from build123d import *
from OCP.BRepFilletAPI import BRepFilletAPI_MakeChamfer

# Parameters (mm, degrees)
EXTRUDE_1_DEPTH     = 60
FILLET_1_R          = 5
CUT_EXTRUDE_1_DEPTH = 5.9
CHAMFER_1_SIZE      = 0.5
CHAMFER_1_SIZE2     = 0.355637567
CHAMFER_1_SIZE2_2   = 0.356604189
SKETCH_6_R          = 2.85
CUT_EXTRUDE_2_DEPTH = 0.1
SKETCH_7_R          = 2.5
CUT_EXTRUDE_3_DEPTH = 75.215901261


with BuildPart() as part:
    # 草图1 → 凸台-拉伸1 (new body)
    with BuildSketch(Plane.XY):
        Polygon((0, 0), (42, 0), (42, 10), (40.535898385, 12), (40, 10), (38.535898385, 12), (38, 10), (36.535898385, 12), (36, 10), (34.535898385, 12), (34, 10), (32.535898385, 12), (32, 10), (30.535898385, 12), (30, 10), (28.535898385, 12), (28, 10), (26.535898385, 12), (26, 10), (24.535898385, 12), (24, 10), (22.535898385, 12), (22, 10), (20.535898385, 12), (20, 10), (18.535898385, 12), (18, 10), (16.535898385, 12), (16, 10), (14.535898385, 12), (14, 10), (12.535898385, 12), (12, 10), (10.535898385, 12), (10, 10), (8.51763809, 11.931851653), (8, 10), (6, 12), (0, 12), align=None)
    extrude(amount=EXTRUDE_1_DEPTH)

    # 圆角1
    fillet_1_edges = [part.edges().sort_by_distance(p)[0] for p in [
        (42, 5, 0),
        (42, 5, 60),
    ]]
    fillet(fillet_1_edges, radius=FILLET_1_R)

    # 草图2 → 切除-拉伸1 (cut)
    with BuildSketch(Plane.ZY):
        with BuildLine():
            ThreePointArc((32.9, 12), (32.050609665, 9.949390335), (30, 9.1))
            Line((30, 9.1), (30, 0))
            Line((30, 0), (39, 0))
            Line((39, 0), (39, 12))
            Line((39, 12), (32.9, 12))
        make_face()
        with BuildLine():
            Line((30, 0), (30, 9.1))
            ThreePointArc((30, 9.1), (27.949390335, 9.949390335), (27.1, 12))
            Line((27.1, 12), (21, 12))
            Line((21, 12), (21, 0))
            Line((21, 0), (30, 0))
        make_face()
        with BuildLine():
            Line((32.9, 12), (30, 12))
            Line((30, 12), (30, 9.1))
            ThreePointArc((30, 9.1), (32.050609665, 9.949390335), (32.9, 12))
        make_face()
        with BuildLine():
            Line((30, 9.1), (30, 12))
            Line((30, 12), (27.1, 12))
            ThreePointArc((27.1, 12), (27.949390335, 9.949390335), (30, 9.1))
        make_face()
    extrude(amount=-CUT_EXTRUDE_1_DEPTH, mode=Mode.SUBTRACT)

    # 倒角1: one chamfer whose edges measure the first distance from different faces: ONE call of the kernel's chamfer builder (chamfer() names one face for all edges)
    chamfer_1_edges_1 = [part.edges().sort_by_distance(p)[0] for p in [
        (40.535898385, 12, 30),
    ]]
    chamfer_1_side_1 = [part.faces().sort_by_distance(p)[0] for p in [
        (40.267229154, 10.997312779, 30),
    ]]
    chamfer_1_edges_2 = [part.edges().sort_by_distance(p)[0] for p in [
        (38.535898385, 12, 30),
    ]]
    chamfer_1_side_2 = [part.faces().sort_by_distance(p)[0] for p in [
        (38.267738685, 10.999214377, 30),
    ]]
    chamfer_1_edges_3 = [part.edges().sort_by_distance(p)[0] for p in [
        (36.535898385, 12, 30),
    ]]
    chamfer_1_side_3 = [part.faces().sort_by_distance(p)[0] for p in [
        (36.267949192, 11, 30),
    ]]
    chamfer_1_edges_4 = [part.edges().sort_by_distance(p)[0] for p in [
        (34.535898385, 12, 30),
    ]]
    chamfer_1_side_4 = [part.faces().sort_by_distance(p)[0] for p in [
        (34.267949192, 11, 30),
    ]]
    chamfer_1_edges_5 = [part.edges().sort_by_distance(p)[0] for p in [
        (32.535898385, 12, 30),
    ]]
    chamfer_1_side_5 = [part.faces().sort_by_distance(p)[0] for p in [
        (32.267949192, 11, 30),
    ]]
    chamfer_1_edges_6 = [part.edges().sort_by_distance(p)[0] for p in [
        (30.535898385, 12, 30),
    ]]
    chamfer_1_side_6 = [part.faces().sort_by_distance(p)[0] for p in [
        (31.267949192, 11, 30),
    ]]
    chamfer_1_edges_7 = [part.edges().sort_by_distance(p)[0] for p in [
        (28.535898385, 12, 30),
    ]]
    chamfer_1_side_7 = [part.faces().sort_by_distance(p)[0] for p in [
        (29.267949192, 11, 30),
    ]]
    chamfer_1_edges_8 = [part.edges().sort_by_distance(p)[0] for p in [
        (26.535898385, 12, 30),
    ]]
    chamfer_1_side_8 = [part.faces().sort_by_distance(p)[0] for p in [
        (27.267949192, 11, 30),
    ]]
    chamfer_1_edges_9 = [part.edges().sort_by_distance(p)[0] for p in [
        (24.535898385, 12, 30),
    ]]
    chamfer_1_side_9 = [part.faces().sort_by_distance(p)[0] for p in [
        (25.267949192, 11, 30),
    ]]
    chamfer_1_edges_10 = [part.edges().sort_by_distance(p)[0] for p in [
        (22.535898385, 12, 30),
    ]]
    chamfer_1_side_10 = [part.faces().sort_by_distance(p)[0] for p in [
        (23.267949192, 11, 30),
    ]]
    chamfer_1_edges_11 = [part.edges().sort_by_distance(p)[0] for p in [
        (20.535898385, 12, 30),
    ]]
    chamfer_1_side_11 = [part.faces().sort_by_distance(p)[0] for p in [
        (21.267949192, 11, 30),
    ]]
    chamfer_1_edges_12 = [part.edges().sort_by_distance(p)[0] for p in [
        (18.535898385, 12, 30),
    ]]
    chamfer_1_side_12 = [part.faces().sort_by_distance(p)[0] for p in [
        (19.267949192, 11, 30),
    ]]
    chamfer_1_edges_13 = [part.edges().sort_by_distance(p)[0] for p in [
        (16.535898385, 12, 30),
    ]]
    chamfer_1_side_13 = [part.faces().sort_by_distance(p)[0] for p in [
        (17.267949192, 11, 30),
    ]]
    chamfer_1_edges_14 = [part.edges().sort_by_distance(p)[0] for p in [
        (14.535898385, 12, 30),
    ]]
    chamfer_1_side_14 = [part.faces().sort_by_distance(p)[0] for p in [
        (15.267949192, 11, 30),
    ]]
    chamfer_1_edges_15 = [part.edges().sort_by_distance(p)[0] for p in [
        (12.535898385, 12, 30),
    ]]
    chamfer_1_side_15 = [part.faces().sort_by_distance(p)[0] for p in [
        (13.267949192, 11, 30),
    ]]
    chamfer_1_edges_16 = [part.edges().sort_by_distance(p)[0] for p in [
        (10.535898385, 12, 30),
    ]]
    chamfer_1_side_16 = [part.faces().sort_by_distance(p)[0] for p in [
        (11.267949192, 11, 30),
    ]]
    chamfer_1_edges_17 = [part.edges().sort_by_distance(p)[0] for p in [
        (8.51763809, 11.931851653, 30),
    ]]
    chamfer_1_side_17 = [part.faces().sort_by_distance(p)[0] for p in [
        (9.258819045, 10.965925826, 30),
    ]]
    chamfer_1 = BRepFilletAPI_MakeChamfer(part.part.solid().wrapped)
    for e in chamfer_1_edges_1:
        chamfer_1.Add(CHAMFER_1_SIZE, CHAMFER_1_SIZE2, e.wrapped, chamfer_1_side_1[0].wrapped)  # the first distance lies on this face
    for e in chamfer_1_edges_2:
        chamfer_1.Add(CHAMFER_1_SIZE, CHAMFER_1_SIZE2, e.wrapped, chamfer_1_side_2[0].wrapped)  # the first distance lies on this face
    for e in chamfer_1_edges_3:
        chamfer_1.Add(CHAMFER_1_SIZE, CHAMFER_1_SIZE2, e.wrapped, chamfer_1_side_3[0].wrapped)  # the first distance lies on this face
    for e in chamfer_1_edges_4:
        chamfer_1.Add(CHAMFER_1_SIZE, CHAMFER_1_SIZE2, e.wrapped, chamfer_1_side_4[0].wrapped)  # the first distance lies on this face
    for e in chamfer_1_edges_5:
        chamfer_1.Add(CHAMFER_1_SIZE, CHAMFER_1_SIZE2, e.wrapped, chamfer_1_side_5[0].wrapped)  # the first distance lies on this face
    for e in chamfer_1_edges_6:
        chamfer_1.Add(CHAMFER_1_SIZE, CHAMFER_1_SIZE2, e.wrapped, chamfer_1_side_6[0].wrapped)  # the first distance lies on this face
    for e in chamfer_1_edges_7:
        chamfer_1.Add(CHAMFER_1_SIZE, CHAMFER_1_SIZE2, e.wrapped, chamfer_1_side_7[0].wrapped)  # the first distance lies on this face
    for e in chamfer_1_edges_8:
        chamfer_1.Add(CHAMFER_1_SIZE, CHAMFER_1_SIZE2, e.wrapped, chamfer_1_side_8[0].wrapped)  # the first distance lies on this face
    for e in chamfer_1_edges_9:
        chamfer_1.Add(CHAMFER_1_SIZE, CHAMFER_1_SIZE2, e.wrapped, chamfer_1_side_9[0].wrapped)  # the first distance lies on this face
    for e in chamfer_1_edges_10:
        chamfer_1.Add(CHAMFER_1_SIZE, CHAMFER_1_SIZE2, e.wrapped, chamfer_1_side_10[0].wrapped)  # the first distance lies on this face
    for e in chamfer_1_edges_11:
        chamfer_1.Add(CHAMFER_1_SIZE, CHAMFER_1_SIZE2, e.wrapped, chamfer_1_side_11[0].wrapped)  # the first distance lies on this face
    for e in chamfer_1_edges_12:
        chamfer_1.Add(CHAMFER_1_SIZE, CHAMFER_1_SIZE2, e.wrapped, chamfer_1_side_12[0].wrapped)  # the first distance lies on this face
    for e in chamfer_1_edges_13:
        chamfer_1.Add(CHAMFER_1_SIZE, CHAMFER_1_SIZE2, e.wrapped, chamfer_1_side_13[0].wrapped)  # the first distance lies on this face
    for e in chamfer_1_edges_14:
        chamfer_1.Add(CHAMFER_1_SIZE, CHAMFER_1_SIZE2, e.wrapped, chamfer_1_side_14[0].wrapped)  # the first distance lies on this face
    for e in chamfer_1_edges_15:
        chamfer_1.Add(CHAMFER_1_SIZE, CHAMFER_1_SIZE2, e.wrapped, chamfer_1_side_15[0].wrapped)  # the first distance lies on this face
    for e in chamfer_1_edges_16:
        chamfer_1.Add(CHAMFER_1_SIZE, CHAMFER_1_SIZE2, e.wrapped, chamfer_1_side_16[0].wrapped)  # the first distance lies on this face
    for e in chamfer_1_edges_17:
        chamfer_1.Add(CHAMFER_1_SIZE, CHAMFER_1_SIZE2_2, e.wrapped, chamfer_1_side_17[0].wrapped)  # the first distance lies on this face
    add(Compound.cast(chamfer_1.Shape()), mode=Mode.REPLACE)

    # 草图6 → 切除-拉伸2 (cut)
    with BuildSketch(Plane.ZY.offset(-5.9)):
        with Locations((30, 12)):
            Circle(SKETCH_6_R)
    extrude(amount=-CUT_EXTRUDE_2_DEPTH, mode=Mode.SUBTRACT)

    # 草图7 → 切除-拉伸3 (cut, through all)
    with BuildSketch(Plane.XZ):
        with Locations(Location((12.2, 52, 0), (0, 0, 270))):
            Circle(SKETCH_7_R)
        with Locations(Location((30, 52, 0), (0, 0, 90))):
            Circle(SKETCH_7_R)
        with Locations(Location((30, 8, 0), (0, 0, 270))):
            Circle(SKETCH_7_R)
        with Locations(Location((12.2, 8, 0), (0, 0, 265.411434264))):
            Circle(SKETCH_7_R)
    extrude(amount=-CUT_EXTRUDE_3_DEPTH, mode=Mode.SUBTRACT)


solid = part.part
Could you check a few things on this model? Use its own coordinates, in mm. A direction names the side the tool comes from. Round coordinates to 2 decimals unless told otherwise and drop trailing zeros. Loops run counter-clockwise (first coordinate to the right, second up) from the corner with the lowest first, then second, coordinate; pieces in that order, holes last. Notation, with made-up numbers: (84.5, 51.5) - (130.5, 51.5) arc R24 ccw to (130.5, 74.5) - close; hole circle Ø10 at (12.25, 61.25). An arc over 180 degrees is marked (long way). Write item = value, one per line.
1) Imagine slicing it at A-A (y = 2.5). Please give me the cut outline in (x, z).
Computed:
outline = (0, 0) - (37, 0) arc R5 ccw to (42, 5) - (42, 55) arc R5 ccw to (37, 60) - (0, 60) - (0, 39) - (5.9, 39) - (5.9, 21) - (0, 21) - close; hole circle Ø5 at (12.2, 8); hole circle Ø5 at (12.2, 52); hole circle Ø5 at (30, 8); hole circle Ø5 at (30, 52)
2) Imagine slicing it at B-B (z = 52). Give the number of separate pieces and of enclosed holes in the cut face, and give its area (3 significant figures).
Computed:
separate_pieces = 3
enclosed_holes = 0
area = 358 mm2
3) I'm going to push flat-ended pins straight in: P1, Ø1, axis at y = 6, z = 26.5, coming from the -X side; P2, Ø3, axis at x = 12.2, z = 8, coming from the -Y side; P3, Ø8, axis at x = 30, z = 8, coming from the -Y side; P4, Ø8, axis at x = 12.2, z = 52, coming from the +Y side. Where does each tip first touch, or does it pass through?
Computed:
P1 = 5.9
P2 = through
P3 = 0
P4 = 11.66
4) If we mould it in two halves opening along Z, with no side actions, what happens to faces 1 (the flat face through (3, 12, 10)), 2 (the flat face through (3, 6, 39))? For each: pulls with the +Z half, pulls with the -Z half, needs draft (parallel to the pull), parting line crosses it, or undercut.
Computed:
face_1 = needs draft
face_2 = undercut
5) I need wall thicknesses on line 1 along X through (y, z) = (9, 8); line 2 along Z through (x, y) = (14, 6); line 3 along Z through (x, y) = (12.2, 6.5). Which ranges of each line are inside material? Lowest first, please. Write a range as from..to.
Computed:
line_1 = 0..9.7, 14.7..27.5, 32.5..42
line_2 = 0..6.27, 9.73..50.27, 53.73..60
line_3 = 0..5.5, 10.5..49.5, 54.5..60
6) On a 3-axis mill with a long thin cutter (end or side, diameter ignored), from which of +Z, -Z, +X, -X, +Y, -Y can I reach the whole of each face in a straight line? I mean faces 3 (the flat face through (3, 6, 21)), 4 (the flat face through (42, 5, 30)). Say none if no direction works.
Computed:
face_3 = -X, +Y, -Y
face_4 = +Z, -Z, +X, +Y, -Y
